from build123d import *

# Parameters (mm, degrees)
F0_R     = 9.525
F0_R_2   = 6.35
F1_DEPTH = 6.35
F2_R     = 6.35
F3_DEPTH = 25.4


with BuildPart() as f1:
    # F0 (on Front) → F1 (new body, symmetric)
    with BuildSketch(Plane.XZ):
        with BuildLine():
            ThreePointArc((101.6, 6.35), (99.740128, 10.840128), (95.25, 12.7))
            Line((95.25, 12.7), (-95.25, 12.7))
            ThreePointArc((-95.25, 12.7), (-99.740128, 10.840128), (-101.6, 6.35))
            Line((-101.6, 6.35), (-101.6, -6.35))
            ThreePointArc((-101.6, -6.35), (-99.740128, -10.840128), (-95.25, -12.7))
            Line((-95.25, -12.7), (95.25, -12.7))
            ThreePointArc((95.25, -12.7), (99.740128, -10.840128), (101.6, -6.35))
            Line((101.6, -6.35), (101.6, 6.35))
        make_face()
        with Locations((-88.9, 0)):
            Circle(F0_R, mode=Mode.SUBTRACT)
        Circle(F0_R_2, mode=Mode.SUBTRACT)
    extrude(amount=F1_DEPTH, both=True)

    # F2 (on face) → F3 (join)
    with BuildSketch(Plane.XZ.offset(6.35)):
        with Locations((88.9, 0)):
            Circle(F2_R)
    extrude(amount=-F3_DEPTH)


solid = f1.part
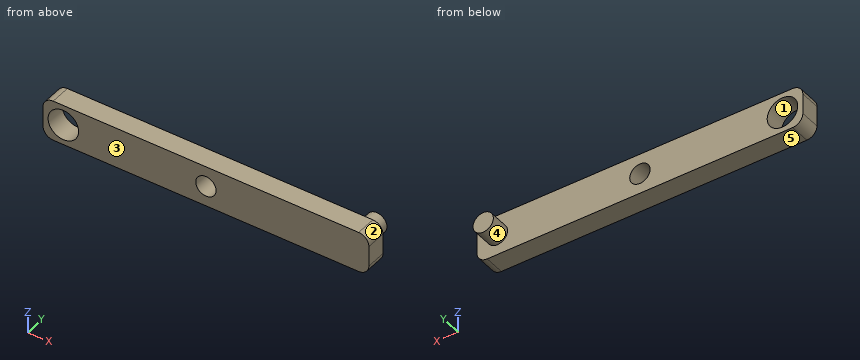
Read the model definition and answer for the solid it produces. Units are mm, in the model's axes. Face numbers are marked on the shaded views. A direction names the side the tool comes from. Coordinates: 2 decimals unless noted, no trailing zeros. Loops run counter-clockwise (first coordinate to the right, second up) from the corner with the lowest first, then second, coordinate; pieces in that order, holes last.
Q1. The part is cut by section A-A on y = 1.25. Write down the section's boundary in (x, z) (3 decimals), and give its area (3 significant figures).
Q2. Which of the six approach directions +Z, -Z, +X, -X, +Y, -Y give full straight-line access (tool end or side, diameter ignored) to the marked faces 4 and 5?
Q3. The part is cut by section C-C on x = 0. Write down the section's boundary in (y, z).
Q4. The mould has two halves that part along Z. Classify the marked faces 1, 2 and 3: +Z half, -Z half, draft (parallel to the pull), parting line (faces both ways), or undercut.
Q5. Each of these flat-tipped pins is pushed along its axis until it touches: pin 1 Ø8 at (x, z) = (68.5, -10) entering from +Y; pin 2 Ø11.5 at (x, z) = (0, 0) entering from -Y; pin 3 Ø3 at (y, z) = (12, -5) entering from -X. Where does it stop, or does it pass through?
Q6. The part is cut by section D-D on x = 88.9. Write down the section's boundary in (y, z), and give its area (3 significant figures).
Q7. Consider probe 1 along X at (y, z) = (2.25, -0.25); probe 2 along Z at (x, y) = (-88.9, -1) (3 decimals); probe 3 along Z at (x, y) = (0, 2.25). Determine where each line is inside the solid, lowest interval first.
Q8. The part is cut by section B-B on z = 0. Write down the section's boundary in (x, y) (3 decimals).
Results below:
1. outline: (-101.6, -6.35) arc R6.35 ccw to (-95.25, -12.7) - (95.25, -12.7) arc R6.35 ccw to (101.6, -6.35) - (101.6, 6.35) arc R6.35 ccw to (95.25, 12.7) - (-95.25, 12.7) arc R6.35 ccw to (-101.6, 6.35) - close; hole circle Ø19.05 at (-88.9, 0); hole circle Ø12.7 at (0, 0)
1. area: 4,710 mm2
2. face 4: +Y
2. face 5: -Z, +X, -X, +Y, -Y
3. outline: (-6.35, -12.7) - (6.35, -12.7) - (6.35, -6.35) - (-6.35, -6.35) - close; (-6.35, 6.35) - (6.35, 6.35) - (6.35, 12.7) - (-6.35, 12.7) - close
4. face 1: undercut
4. face 2: +Z half
4. face 3: draft
5. pin 1: stops at y = 6.35
5. pin 2: passes through
5. pin 3: stops at x = 83.6
6. outline: (-6.35, -12.7) - (6.35, -12.7) - (6.35, -6.35) - (19.05, -6.35) - (19.05, 6.35) - (6.35, 6.35) - (6.35, 12.7) - (-6.35, 12.7) - close
6. area: 484 mm2
7. probe 1: x = -101.6 to -98.42, -79.38 to -6.35, 6.35 to 101.6
7. probe 2: z = -12.7 to -9.525, 9.525 to 12.7
7. probe 3: z = -12.7 to -6.35, 6.35 to 12.7
8. outline: (-101.6, -6.35) - (-98.425, -6.35) - (-98.425, 6.35) - (-101.6, 6.35) - close; (-79.375, -6.35) - (-6.35, -6.35) - (-6.35, 6.35) - (-79.375, 6.35) - close; (6.35, -6.35) - (101.6, -6.35) - (101.6, 6.35) - (95.25, 6.35) - (95.25, 19.05) - (82.55, 19.05) - (82.55, 6.35) - (6.35, 6.35) - close
